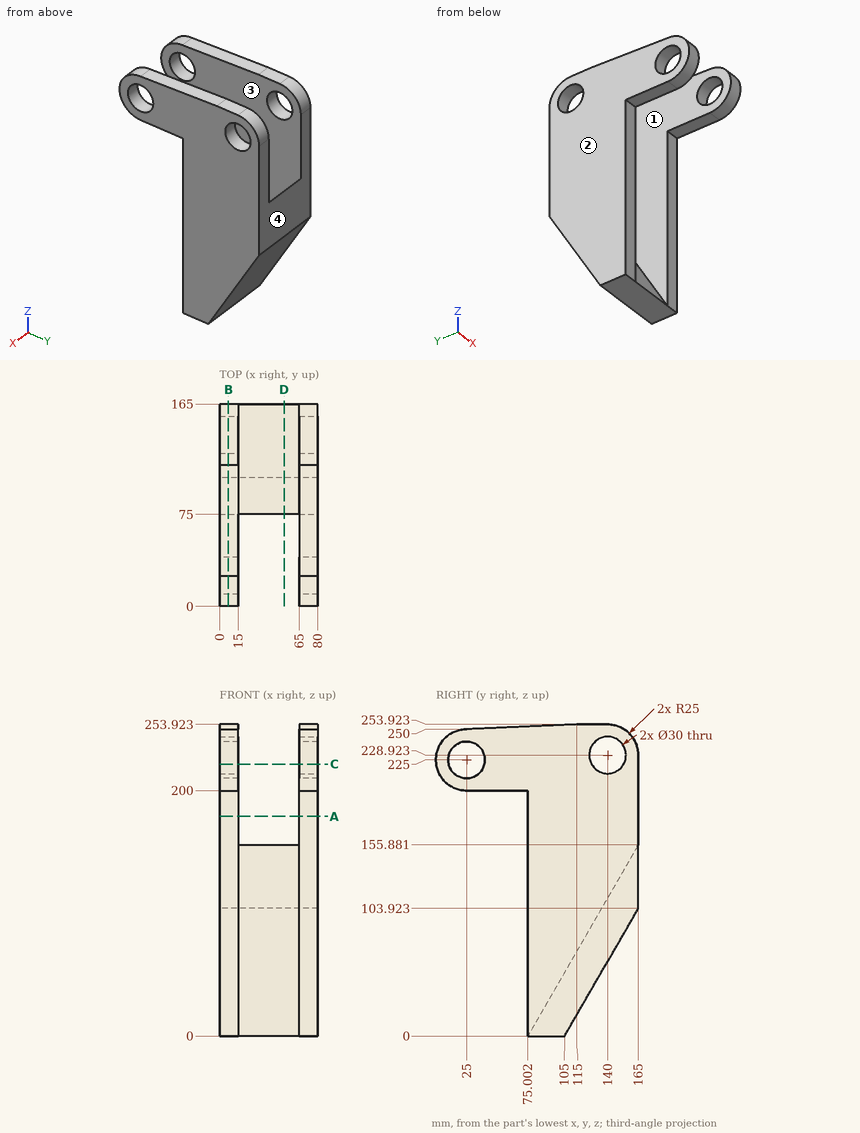
Could you check a few things on this drawing? It's one solid part, dimensions in mm from its lowest x, y, z. Coordinates: 2 decimals unless noted, no trailing zeros. Loops run counter-clockwise (first coordinate to the right, second up) from the corner with the lowest first, then second, coordinate; pieces in that order, holes last.
1. I need wall thicknesses on L1, parallel to X at y = 111.5, z = 192; L2, parallel to Z at x = 75, y = 25; L3, parallel to Z at x = 75, y = 140 (1 decimal). Which ranges of each line are inside material? Lowest first, please.
2. Imagine slicing it at A-A (z = 179). Please give me the cut outline in (x, y), and give its area (3 significant figures).
3. Imagine slicing it at C-C (z = 221.5). Please give me the cut outline in (x, y) (1 decimal).
4. For P1, Ø24, axis at y = 25, z = 225, coming from the -X side; P2, Ø7.5, axis at x = 70, z = 59.5, coming from the -Y side; P3, Ø4.5, axis at x = 11, y = 43, coming from the -Z side; P4, Ø12, axis at x = 54, y = 136, coming from the +Z side (1 decimal), each with a flat end and sliding along its axis, tell me the tip position at first contact or that it passes through.
5. Imagine slicing it at D-D (x = 52.5). Please give me the cut outline in (y, z), and give its area (3 significant figures).
6. Imagine slicing it at B-B (x = 7). Please give me the cut outline in (y, z), and give its area (3 significant figures).
7. We'd pull the mould along X, two halves only. Please class the marked faces 1, 2, 3 and 4: released by +X, released by -X, zero draft, split by the parting line, or undercut.
Computed values:
1. L1: x = 0 to 15, 65 to 80
1. L2: z = 200 to 210, 240 to 250
1. L3: z = 60.6 to 213.9, 243.9 to 253.9
2. outline: (0, 75) - (15, 75) - (15, 165) - (0, 165) - close; (65, 75) - (80, 75) - (80, 165) - (65, 165) - close
2. area: 2,700 mm2
3. outline: (0, 0.2) - (15, 0.2) - (15, 10.4) - (0, 10.4) - close; (0, 39.6) - (15, 39.6) - (15, 127) - (0, 127) - close; (0, 153) - (15, 153) - (15, 165) - (0, 165) - close; (65, 0.2) - (80, 0.2) - (80, 10.4) - (65, 10.4) - close; (65, 39.6) - (80, 39.6) - (80, 127) - (65, 127) - close; (65, 153) - (80, 153) - (80, 165) - (65, 165) - close
4. P1: passes through
4. P2: stops at y = 75
4. P3: stops at z = 200
4. P4: stops at z = 116
5. outline: (75, 0) - (105, 0) - (165, 103.92) - (165, 155.88) - close
5. area: 3,900 mm2
6. outline: (25, 200) - (75, 200) - (75, 0) - (105, 0) - (165, 103.92) - (165, 228.92) arc R25 ccw to (140, 253.92) - (115, 253.92) - (25, 250) arc R25 ccw to start; hole circle Ø30 at (25, 225); hole circle Ø30 at (140, 228.92)
6. area: 21,700 mm2
7. face 1: undercut
7. face 2: released by -X
7. face 3: undercut
7. face 4: zero draft
